Here's how the part is built. I have some questions about the finished solid (model axes, mm). A direction names the side the tool comes from. Round coordinates to 2 decimals unless told otherwise and drop trailing zeros. Write each loop counter-clockwise with the first axis right and the second up, starting at its lowest first coordinate (ties: lowest second). Pieces come first, ordered by that corner, then holes. Notation, with made-up numbers: (-35, 68.25) - (-1, 68.25) arc R23 ccw to (-1, 101.25) - close; hole circle Ø6 at (-38.75, 89). An arc over 180 degrees is marked (long way). Write item = value, one per line. Start each with the question number.
Item 1: Thinking about a two-plate mould opening in Y: for faces 3 (the face through (139.7, 46, 47)), 4 (the face through (107, 0, 24)), 5 (the face through (107, 92.71, 24)), which applies, pulls with the +Y half, pulls with the -Y half, needs draft (parallel to the pull), parting line crosses it, or undercut?
Item 2: If we section it at A-A (x = 50.8): Please give me the cut outline in (y, z), and give its area (3 significant figures).
Item 3: For P1, Ø13, axis at x = 149.35, y = 46.63, coming from the +Z side, with a flat end and sliding along its axis, tell me the tip position at first contact or that it passes through.
Item 4: If I drill on line 1 along X through (y, z) = (33, 4); line 2 along Z through (x, y) = (142, 5); line 3 along Y through (x, z) = (152.5, 36.5), over which ranges is the centre line in solid material (lowest first)? Write a range as [from, to].
Item 5: Which directions (+Z, -Z, +X, -X, +Y, -Y) give clear straight access to the entire face, cutting with the end or side of a thin tool? Please do faces 1 (the face through (178.33, 46.22, 43.18)), 2 (the face through (38.224, 1.449, 1.528)).
```python
from build123d import *

# Parameters (mm, degrees)
F0_W         = 215.9
F0_H         = 92.71
F1_DEPTH     = 49.53
F3_DEPTH     = 76.2
F5_DEPTH     = 92.71
F6_R         = 5.08
F7_R         = 6.35
F8_DEPTH     = 92.7110001
F9_T1_DEPTH  = 26.67
F9_S5_W      = 5.08
F9_S5_H      = 5.08
F9_T6_DEPTH  = 5.08
F9_S11_W     = 5.08
F9_S11_H     = 5.08
F9_T12_DEPTH = 5.08
F10_R        = 5.588
F11_DEPTH    = 49.5310001


# Not quite as in the source:
# - a fillet or chamfer that OpenCascade refuses, or shapes differently, is made with other operations: its cross-section is extruded or revolved along the edge and cut away or added


with BuildPart() as f1:
    # F0 (on Top) → F1 (new body)
    with BuildSketch(Plane.XY):
        with Locations((107.95, 46.355)):
            Rectangle(F0_W, F0_H)
    extrude(amount=F1_DEPTH)

    # F2 (on face) → F3 (cut)
    with BuildSketch(Plane.YZ.offset(215.9)):
        with BuildLine():
            Line((52.705, 49.53), (40.005, 49.53))
            ThreePointArc((40.005, 49.53), (46.355, 43.18), (52.705, 49.53))
        make_face()
    extrude(amount=-F3_DEPTH, mode=Mode.SUBTRACT)

    # F4 (on face) → F5 (cut, through all)
    with BuildSketch(Plane.XZ):
        with BuildLine():
            Line((19.05, 0), (31.75, 0))
            ThreePointArc((31.75, 0), (25.4, 6.35), (19.05, 0))
        make_face()
    extrude(amount=-F5_DEPTH, mode=Mode.SUBTRACT)

    # F6
    f6_edges = [f1.edges().sort_by_distance(p)[0] for p in [
        (107.95, 0, 49.53),
        (215.9, 20.0025, 49.53),
        (107.95, 92.71, 49.53),
        (215.9, 72.7075, 49.53),
        (0, 92.71, 24.765),
        (0, 46.355, 49.53),
        (0, 0, 24.765),
        (0, 46.355, 0),
        (123.825, 0, 0),
        (123.825, 92.71, 0),
        (215.9, 46.355, 0),
        (215.9, 92.71, 24.765),
        (215.9, 0, 24.765),
    ]]
    fillet(f6_edges, radius=F6_R)

    # F7 (on Front) → F8 (cut, through all)
    with BuildSketch(Plane.XZ):
        with Locations((50.8, 0)):
            Circle(F7_R)
    extrude(amount=-F8_DEPTH, mode=Mode.SUBTRACT)

    # F9: fillet of radius 5.08 on 2 edges, made by hand

    # F9_s2 → F9_t1 (cut)
    with BuildSketch(Plane.YZ.offset(5.08)):
        with BuildLine():
            ThreePointArc((5.08, 0), (1.4878975516, 1.4878975516), (0, 5.08))
            Line((0, 5.08), (0, 0))
            Line((0, 0), (5.08, 0))
        make_face()
        with BuildLine():
            ThreePointArc((92.71, 5.08), (91.2221024484, 1.4878975516), (87.63, 0))
            Line((87.63, 0), (92.71, 0))
            Line((92.71, 0), (92.71, 5.08))
        make_face()
    extrude(amount=F9_T1_DEPTH, mode=Mode.SUBTRACT)


with BuildPart() as f9_tool4:
    # F9_s5 → F9_t6 (new body)
    with BuildSketch(Plane.XZ.offset(-87.63)):
        with Locations((2.54, 2.54)):
            Rectangle(F9_S5_W, F9_S5_H)
    extrude(amount=-F9_T6_DEPTH)

    # F9_s7 → F9_t8 (revolve, cut)
    with BuildSketch(Plane(origin=(5.08, 87.63, 5.08), x_dir=(0.7071067812, 0, 0.7071067812), z_dir=(-0.7071067812, 0, 0.7071067812))):
        with BuildLine():
            ThreePointArc((0, -5.08), (5.08, 0), (0, 5.08))
            Line((0, 5.08), (0, -5.08))
        make_face()
    revolve(axis=Axis((5.08, 87.63, 5.08), (0, 1, 0)), mode=Mode.SUBTRACT)


with BuildPart() as f1_1:
    add(f1.part)

    # F9_t3: cut F9_tool4
    add(f9_tool4.part, mode=Mode.SUBTRACT)


with BuildPart() as f9_tool10:
    # F9_s11 → F9_t12 (new body)
    with BuildSketch(Plane.XY.offset(5.08)):
        with Locations((2.54, 2.54)):
            Rectangle(F9_S11_W, F9_S11_H)
    extrude(amount=-F9_T12_DEPTH)

    # F9_s13 → F9_t14 (revolve, cut)
    with BuildSketch(Plane(origin=(5.08, 5.08, 5.08), x_dir=(0.7071067812, 0.7071067812, 0), z_dir=(-0.7071067812, 0.7071067812, 0))):
        with BuildLine():
            ThreePointArc((0, -5.08), (5.08, 0), (0, 5.08))
            Line((0, 5.08), (0, -5.08))
        make_face()
    revolve(axis=Axis((5.08, 5.08, 5.08), (0, 0, -1)), mode=Mode.SUBTRACT)


with BuildPart() as f1_2:
    add(f1_1.part)

    # F9_t9: cut F9_tool10
    add(f9_tool10.part, mode=Mode.SUBTRACT)

    # F10 (on face) → F11 (cut, through all)
    with BuildSketch(Plane.XY.offset(49.53)):
        with Locations((149.3525841786, 46.6338395569)):
            Circle(F10_R)
    extrude(amount=-F11_DEPTH, mode=Mode.SUBTRACT)


solid = f1_2.part
```
Reply:
q1.face_3 = undercut
q1.face_4 = pulls with the -Y half
q1.face_5 = pulls with the +Y half
q2.outline = (0, 6.35) - (92.71, 6.35) - (92.71, 44.45) arc R5.08 ccw to (87.63, 49.53) - (5.08, 49.53) arc R5.08 ccw to (0, 44.45) - close
q2.area = 3,990 mm2
q3.P1 = 49.53
q4.line_1 = [0.12, 20.47], [30.33, 45.87], [55.73, 215.78]
q4.line_2 = [0, 49.53]
q4.line_3 = [0, 42.02], [51.25, 92.71]
q5.face_1 = +Z, +X
q5.face_2 = -Z, +X, -X, -Y
